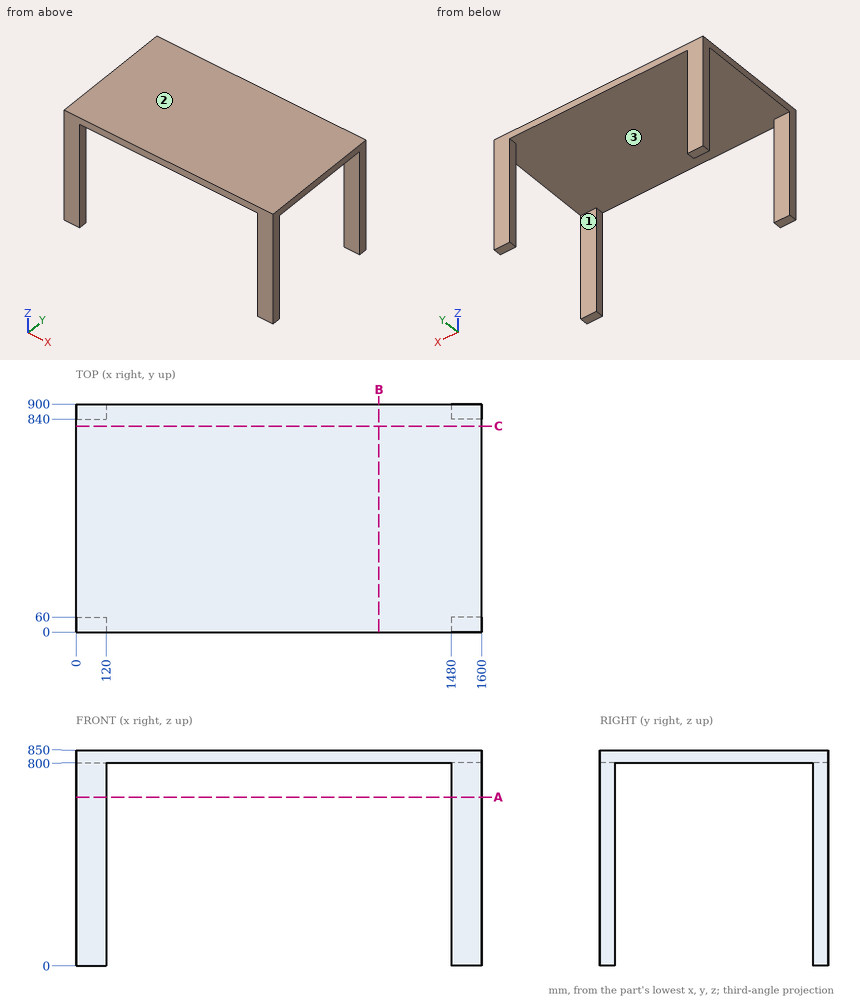
Geometry check sheet. Reference: drawing and pictorial views, mm from the part's lowest x, y, z. Round coordinates to 2 decimals unless told otherwise and drop trailing zeros. Order: outer loops, then holes, each group sorted by start corner. A loop starts at its lowest first (then second) coordinate and runs counter-clockwise, first axis right, second up. Notation, with made-up numbers: (49, 32) -> (105, 32) arc R13 ccw to (105, 51) -> close; hole circle Ø9 at (-13.5, -6.75). An arc over 180 degrees is marked (long way). One line per item, written item: value. Start each with the question number.
Q1. Cross-section at A-A (z = 665.5). Record the boundary of the cut face in (x, y), and give its area (3 significant figures).
Q2. Cross-section at C-C (y = 813). Record the boundary of the cut face in (x, z).
Q3. Gauge pin test, flat end, axial feed: pin 1 Ø4 at (x, y) = (1428.5, 504.5) entering from -Z. Record the tip position at first contact, or that the pin passes through.
Q4. Mould release check, pull along Y, two halves, no side actions. Record for the marked faces 1, 2 and 3: pulls with the +Y half, pulls with the -Y half, needs draft (parallel to the pull), parting line crosses it, or undercut.
Q5. Thickness scan on line 1 (Y direction, x = 1484.5, z = 131); line 2 (Z direction, x = 1147.5, y = 279); line 3 (X direction, y = 58, z = 477.5). Record the ranges inside material, lowest first.
Q6. Cross-section at B-B (x = 1194.5). Record the boundary of the cut face in (y, z).
Completed:
1. outline: (0, 0) -> (120, 0) -> (120, 60) -> (0, 60) -> close; (0, 840) -> (120, 840) -> (120, 900) -> (0, 900) -> close; (1480, 0) -> (1600, 0) -> (1600, 60) -> (1480, 60) -> close; (1480, 840) -> (1600, 840) -> (1600, 900) -> (1480, 900) -> close
1. area: 28,800 mm²
2. outline: (0, 800) -> (1600, 800) -> (1600, 850) -> (0, 850) -> close
3. pin 1: stops at z = 800
4. face 1: undercut
4. face 2: needs draft
4. face 3: undercut
5. line 1: y = 0 to 60, 840 to 900
5. line 2: z = 800 to 850
5. line 3: x = 0 to 120, 1480 to 1600
6. outline: (0, 800) -> (900, 800) -> (900, 850) -> (0, 850) -> close
